Could you check a few things on this model? Use its own coordinates, in mm. A direction names the side the tool comes from. Give positions to 0.01 mm unless a question says otherwise; leave off trailing zeros. Loops run counter-clockwise (first coordinate to the right, second up) from the corner with the lowest first, then second, coordinate; pieces in that order, holes last. Notation, with made-up numbers: (52, -31.75) - (67, -31.75) arc R21 cw to (67, -2.75) - close; hole circle Ø5 at (44.5, 28.25). An arc over 180 degrees is marked (long way). Answer in a Markdown table with one row per item. Add a question column.
Autodesk Inventor part; units mm, degrees
ref_plane "YZ Plane" through (0, 0, 0) normal (1, 0, 0) x (0, 1, 0)
ref_plane "XZ Plane" through (0, 0, 0) normal (0, 1, 0) x (-1, 0, 0)
ref_plane "XY Plane" through (0, 0, 0) normal (0, 0, 1) x (1, 0, 0)
sketch "Sketch1" plane through (0, 0, 0) normal (0, 0, 1) x (1, 0, 0)
  line L0 (-42, 30) -> (42, 30)
  line L1 (44, 28) -> (44, -28)
  line L2 (42, -30) -> (-42, -30)
  line L3 (-44, -28) -> (-44, 28)
  line L4 (-44, 30) -> (44, -30) construction
  line L5 (44, 30) -> (-44, -30) construction
  line L6 (-41.0667, 28) -> (41.0667, 28)
  line L7 (42.5, 26.5) -> (42.5, -26.5)
  line L8 (41.0667, -28) -> (-41.0667, -28)
  line L9 (-42.5, -26.5) -> (-42.5, 26.5)
  line L10 (-42.5, 28) -> (42.5, -28) construction
  line L11 (42.5, 28) -> (-42.5, -28) construction
  arc A0 (-41, 28) -> (-42.5, 26.5) centre (-41, 26.5) ccw
  arc A1 (42.5, 26.5) -> (41, 28) centre (41, 26.5) ccw
  arc A2 (41, -28) -> (42.5, -26.5) centre (41, -26.5) ccw
  arc A3 (-42.5, -26.5) -> (-41, -28) centre (-41, -26.5) ccw
  arc A4 (-44, -28) -> (-42, -30) centre (-42, -28) ccw
  arc A5 (-42, 30) -> (-44, 28) centre (-42, 28) ccw
  arc A6 (44, 28) -> (42, 30) centre (42, 28) ccw
  arc A7 (42, -30) -> (44, -28) centre (42, -28) ccw
  point P0 (0, 0)
  dimension "d0" = 88
  dimension "d1" = 60
  dimension "d2" = 85
  dimension "d3" = 56
  dimension "d4" = 3
  dimension "d5" = 3
  dimension "d6" = 2
extrude "Extrusion1" add sketch "Sketch1" against normal blind 2 contours L0 A6 L1 A7 L2 A4 L3 A5 | L6 A1 L7 A2 L8 A3 L9 A0
extrude "Extrusion2" add sketch "Sketch1" along normal blind 9.5
sketch "Sketch2" plane through (44, -28, -2) normal (1, 0, 0) x (0, 0, -1)
  point P0 (-2, 28)
sketch "Sketch3" plane through (44, -28, -2) normal (1, 0, 0) x (0, 0, -1)
  line L0 (0, -2) -> (-11.5, -2)
  line L1 (-11.5, -2) -> (-11.5, 2)
  line L2 (-11.5, 1.5) -> (-11.5, 54.5)
  line L3 (-11.5, 2) -> (-6.5, 2)
  line L4 (-6.5, 2) -> (-6.5, 58)
  line L5 (0, 58) -> (-11.5, 58)
  line L6 (-11.5, 58) -> (-11.5, 54)
  line L7 (-11.5, 54) -> (-6.5, 54)
  line L8 (-11.5, 54) -> (-11.5, 2)
  point P0 (-2, 28)
  dimension "d11" = 4
  dimension "d12" = 5
  dimension "d13" = 4
  dimension "d14" = 53
extrude "Extrusion3" cut sketch "Sketch3" against normal mid plane 9.5 contours L2 L7 L4 L3
sketch "Sketch4" plane through (-42, -30, -2) normal (0, -1, 0) x (1, 0, 0)
  line L0 (84, 0) -> (86, 0)
  circle A0 centre (53.5, 9) radius 3.5
  line L1 (18.9875, 0) -> (24.4875, 0)
  line L2 (-2, 0) -> (-2, 11.5)
  line L3 (43, 5.8) -> (43, 11.5)
  line L4 (35, 5.8) -> (35, 11.5)
  line L5 (30, 5.8) -> (30, 11.5)
  line L6 (22, 5.8) -> (22, 11.5)
  line L7 (17, 5.8) -> (17, 11.5)
  line L8 (7, 5.8) -> (7, 11.5)
  line L9 (83, 11.5) -> (1, 11.5)
  line L10 (17, 11.5) -> (7, 11.5)
  line L11 (22, 11.5) -> (30, 11.5)
  line L12 (35, 11.5) -> (43, 11.5)
  line L13 (86, 0) -> (86, 11.5)
  line L14 (84, 0) -> (0, 0)
  line L15 (7, 5.8) -> (17, 5.8)
  line L16 (22, 5.8) -> (30, 5.8)
  line L17 (35, 5.8) -> (43, 5.8)
  point P0 (42, 2)
  point P1 (55.9495, 11.5)
  point P2 (51.0505, 11.5)
  dimension "d19" = 7
  dimension "d22" = 8
  dimension "d23" = 5
  dimension "d24" = 8
  dimension "d25" = 5
  dimension "d26" = 10
  dimension "d27" = 32.5
  dimension "d28" = 9
  dimension "d29" = 5.8
  dimension "d38" = 10.5
extrude "Extrusion4" cut sketch "Sketch4" against normal blind 9.5 contours A0 L9 | L7 L15 L8 L9 | L5 L16 L6 L9 | L3 L17 L4 L9 picked at (52.2452, 9.1659)
sketch "Sketch5" plane through (0, 0, -2) normal (0, 0, -1) x (-1, 0, 0)
  line L0 (44, -8) -> (34, -8)
  line L1 (34, -8) -> (34, 8)
  line L2 (34, 8) -> (44, 8)
  line L3 (44, 8) -> (44, -8)
  line L4 (-42, -30) -> (42, -30)
  line L5 (42, 30) -> (-42, 30)
  line L6 (44, -28) -> (44, 28)
  point P0 (0, 0)
  dimension "d32" = 22
  dimension "d33" = 22
  dimension "d34" = 0
  dimension "d35" = 10
extrude "Extrusion5" cut sketch "Sketch5" against normal blind 15
properties part number "Pi 4 Case - Back Panel"
(1) Please list where these lines run through material, in increasing order: line 1 (Y direction, x = -24.5, z = 6); line 2 (X direction, y = -29.25, z = 7); line 3 (X direction, y = -28.65, z = 7).
(2) I want a section at C-C on y = -7. Please give me the cut outline in (x, z).
(3) On a 3-axis mill with a long thin cutter (end or side, diameter ignored), from which of +Z, -Z, +X, -X, +Y, -Y can I reach the whole of each face in a straight line? I mean faces 5 (the flat face through (-34, 0, -1)), 6 (the flat face through (1, -29, 7)), 7 (the flat face through (-1, 28, 5)). Say none if no direction works.
(4) For pin 1 Ø0.6 at (y, z) = (2.5, -1.5) entering from -X; pin 2 Ø1.6 at (y, z) = (-29.5, 7) entering from +X; pin 3 Ø1 at (x, y) = (-3, -28.5) entering from +Z, each with a flat end and sliding along its axis, tell me the tip position at first contact or that it passes through.
(5) I want a section at B-B on z = -1. Please give me the cut outline in (x, y), then the cut area to 3 significant figures.
(6) We'd pull the mould along X, two halves only. Please class faces 1 (the flat face through (-7, -29, 7)), 2 (the cylindrical face through (43.43, -29.4, 3.67)), 3 (the flat face through (-42.5, -17, 5)), 4 (the flat face through (-1, 30, 4)): pulls with the +X half, pulls with the -X half, needs draft (parallel to the pull), parting line crosses it, or undercut.
(7) I want a section at D-D on x = 11.5. Please give me the cut outline in (y, z).
(8) I want a section at A-A on x = -32.5. Please give me the cut outline in (y, z).
Reported:
| question | item | result |
|---|---|---|
| 1 | line 1 | -30 to -28, 28 to 30 |
| 1 | line 2 | -43.56 to -35, -25 to -20, -12 to -7, 1 to 8, 15 to 43.56 |
| 1 | line 3 | -43.89 to -35, -25 to -20, -12 to -7, 1 to 8, 15 to 43.89 |
| 2 | outline | (-34, -2) - (44, -2) - (44, 4.5) - (42.5, 4.5) - (42.5, 0) - (-34, 0) - close |
| 3 | face 5 | +Z, -Z, -X |
| 3 | face 6 | +Z, -Y |
| 3 | face 7 | +Z |
| 4 | pin 1 | x = -34 |
| 4 | pin 2 | x = 43.87 |
| 4 | pin 3 | z = 3.8 |
| 5 | outline | (-44, -28) arc R2 ccw to (-42, -30) - (42, -30) arc R2 ccw to (44, -28) - (44, 28) arc R2 ccw to (42, 30) - (-42, 30) arc R2 ccw to (-44, 28) - (-44, 8) - (-34, 8) - (-34, -8) - (-44, -8) - close |
| 5 | area | 5,120 mm² |
| 6 | face 1 | undercut |
| 6 | face 2 | pulls with the +X half |
| 6 | face 3 | undercut |
| 6 | face 4 | needs draft |
| 7 | outline | (-30, -2) - (30, -2) - (30, 9.5) - (28, 9.5) - (28, 0) - (-28, 0) - (-28, 3.5) - (-30, 3.5) - close |
| 8 | outline | (-30, -2) - (30, -2) - (30, 9.5) - (28, 9.5) - (28, 0) - (-28, 0) - (-28, 3.8) - (-30, 3.8) - close |
